Input: dimensioned drawing with shaded views. Units: mm. Origin: part minimum x, y, z. A direction names the side the tool comes from. Give positions to 0.01 mm unless a question says otherwise; leave off trailing zeros. Loops run counter-clockwise (first coordinate to the right, second up) from the corner with the lowest first, then second, coordinate; pieces in that order, holes last. Notation, with made-up numbers: (-28, 61.25) -> (8, 61.25) arc R21 ccw to (8, 86.25) -> close; hole circle Ø11 at (16.25, -14.75). An arc over 180 degrees is marked (long way). Answer as a JSON object with one key per item and string values.
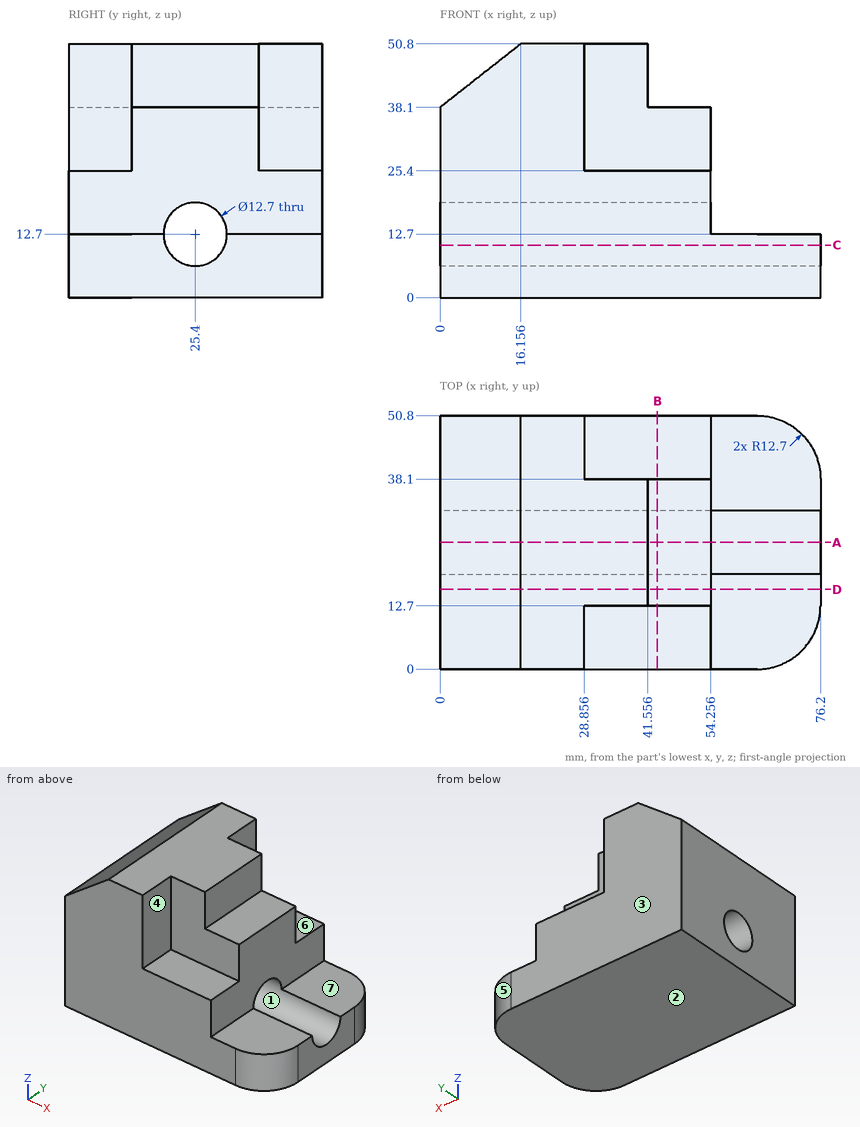
Q1. Draft query along Y for the marked faces 1, 2 and 3. Return one class per face: +Y half, -Y half, draft (parallel to the pull), parting line (faces both ways), or undercut.
Evaluation:
{"face 1": "undercut", "face 2": "draft", "face 3": "+Y half"}
Q2. Ray query, line 1 along Z through (x, y) = (50.5, 25.4); line 2 along Y through (x, z) = (38, 12.7); line 3 along X through (y, z) = (38.5, 24.5). Return the intervals inside material, ascending.
Evaluation:
{"line 1": "z = 0 to 6.35, 19.05 to 38.1", "line 2": "y = 0 to 19.05, 31.75 to 50.8", "line 3": "x = 0 to 54.26"}
Q3. Section A-A, the plane y = 25.4. Return the cut outline in (x, z), then the cut area to 3 significant figures.
Evaluation:
{"outline": "(0, 0) -> (76.2, 0) -> (76.2, 6.35) -> (0, 6.35) -> close; (0, 19.05) -> (54.26, 19.05) -> (54.26, 38.1) -> (41.56, 38.1) -> (41.56, 50.8) -> (16.16, 50.8) -> (0, 38.1) -> close", "area": "1,940 mm2"}
Q4. Access query for the marked faces 4, 5, 6 and 7. Directions: +Z, -Z, +X, -X, +Y, -Y. A direction counts if a zero-diameter tool reaches every point of the face in a straight line with its end or side. Return the directions, or none.
Evaluation:
{"face 4": "+Z, +X, -Y", "face 5": "+Z, -Z, +X, +Y", "face 6": "+Z, +X, +Y", "face 7": "+Z, +X, +Y, -Y"}
Q5. Section D-D, the plane y = 16. Return the cut outline in (x, z).
Evaluation:
{"outline": "(0, 0) -> (76.2, 0) -> (76.2, 12.7) -> (54.26, 12.7) -> (54.26, 38.1) -> (41.56, 38.1) -> (41.56, 50.8) -> (16.16, 50.8) -> (0, 38.1) -> close"}
Q6. Section C-C, the plane z = 10.5. Return the cut outline in (x, y).
Evaluation:
{"outline": "(0, 0) -> (63.5, 0) arc R12.7 ccw to (76.2, 12.7) -> (76.2, 19.44) -> (0, 19.44) -> close; (0, 31.36) -> (76.2, 31.36) -> (76.2, 38.1) arc R12.7 ccw to (63.5, 50.8) -> (0, 50.8) -> close"}
Q7. Pin query (flat end, axial travel): pin 1 (10 mm diameter, centred on x = 38, y = 3.5, fed in from +Z); pin 2 (5 mm diameter, centred on x = 53, y = 12, fed in from +Z); pin 3 (12.5 mm diameter, centred on x = 38, z = 40.5, fed in from -Y); pin 4 (14.5 mm diameter, centred on y = 25.4, z = 12.7, fed in from +X). Return the tip coordinate at first contact, or that it passes through.
Evaluation:
{"pin 1": "stops at z = 25.4", "pin 2": "stops at z = 38.1", "pin 3": "stops at y = 12.7", "pin 4": "stops at x = 76.2"}
Q8. Section B-B, the plane x = 43.5. Return the cut outline in (y, z), then the cut area to 3 significant figures.
Evaluation:
{"outline": "(0, 0) -> (50.8, 0) -> (50.8, 25.4) -> (38.1, 25.4) -> (38.1, 38.1) -> (12.7, 38.1) -> (12.7, 25.4) -> (0, 25.4) -> close; hole circle Ø12.7 at (25.4, 12.7)", "area": "1,490 mm2"}
